Source: CAD feature listing. Evaluate the final solid. Frame: model axes, mm. Give positions to 0.01 mm unless a question says otherwise; leave off trailing zeros. Write item = value, one per line.
from build123d import *

# Parameters (mm, degrees)
ESQUISSE1_R                               = 156.21
ESQUISSE1_R_2                             = 142.07
BOSS_EXTRU_1_DEPTH                        = 2
ESQUISSE2_R                               = 5.85
ENL_V_MAT_EXTRU_1_DEPTH                   = 2
CHANFREIN1_SIZE                           = 0.5
R_P_TITION_CIRCULAIRE1_COUNT              = 70
CHANFREIN1_OF_R_P_TITION_CIRCULAIRE1_SIZE = 0.5
INTERSECT4_OUTLINE_R                      = 5.85
INTERSECT4_DEPTH                          = 2


# Read off the part's stored shape, not the designer's step: Intersect4
with BuildPart() as part:
    # Esquisse1 → Boss.-Extru.1 (new body)
    with BuildSketch(Plane(origin=(0, 0, 0), x_dir=(1, 0, 0), z_dir=(0, 1, 0))):
        with Locations(Location((0, 0, 0), (0, 0, 270))):
            Circle(ESQUISSE1_R)
        with Locations(Location((0, 0, 0), (0, 0, 270))):
            Circle(ESQUISSE1_R_2, mode=Mode.SUBTRACT)
    extrude(amount=BOSS_EXTRU_1_DEPTH)

    # Esquisse2 → Enlèv. mat.-Extru.1 (cut)
    with BuildSketch(Plane.XZ):
        with Locations(Location((-138.182447366, 56.110162301, 0), (0, 0, 270))):
            Circle(ESQUISSE2_R)
    enl_v_mat_extru_1 = extrude(amount=-ENL_V_MAT_EXTRU_1_DEPTH, mode=Mode.SUBTRACT)

    # Chanfrein1
    chanfrein1_edges = [part.edges().sort_by_distance(p)[0] for p in [
        (-138.182447366, 0, 61.960162301),
    ]]
    chamfer(chanfrein1_edges, length=CHANFREIN1_SIZE)

    # Répétition circulaire1: Enlèv. mat.-Extru.1 ×70 about axis
    r_p_tition_circulaire1_axis = Axis((0, 0, 0), (0, 1, 0))
    for i in range(1, R_P_TITION_CIRCULAIRE1_COUNT):
        add(enl_v_mat_extru_1.rotate(r_p_tition_circulaire1_axis, i * 360 / R_P_TITION_CIRCULAIRE1_COUNT), mode=Mode.SUBTRACT)

    # Chanfrein1 of Répétition circulaire1
    chanfrein1_of_r_p_tition_circulaire1_edges = [part.edges().sort_by_distance(p)[0] for p in [
        (-132.07209933, 0, 74.097307988),
        (-124.898384407, 0, 85.63786572),
        (-116.719061132, 0, 96.488917711),
        (-107.599984606, 0, 106.563097671),
        (-97.614576272, 0, 115.779294227),
        (-86.843232766, 0, 124.063303983),
        (-75.372678613, 0, 131.348428963),
        (-63.295267971, 0, 137.576013625),
        (-50.708241047, 0, 142.695917119),
        (-37.712941183, 0, 146.666916991),
        (-24.413998891, 0, 149.457041087),
        (-10.918489435, 0, 151.043824968),
        (2.664929277, 0, 151.414492782),
        (16.226891547, 0, 150.56606013),
        (29.658204426, 0, 148.505358094),
        (42.850726883, 0, 145.248978234),
        (55.698240482, 0, 140.823139006),
        (68.097304599, 0, 135.263474666),
        (79.94808926, 0, 128.614748362),
        (91.155178915, 0, 120.930491727),
        (101.628340667, 0, 112.27257388),
        (111.283250778, 0, 102.710703283),
        (120.042173586, 0, 92.321866495),
        (127.834587396, 0, 81.189708324),
        (134.597752274, 0, 69.403858359),
        (140.277215193, 0, 57.059209336),
        (144.827248457, 0, 44.255153109),
        (148.211217874, 0, 31.094780412),
        (150.40187771, 0, 17.684050826),
        (151.381590063, 0, 4.13093966),
        (151.142466863, 0, -9.455431402),
        (149.68643339, 0, -22.965672891),
        (147.02521277, 0, -36.291008285),
        (143.180231586, 0, -49.324149819),
        (138.182447366, 0, -61.960162301),
        (132.07209933, 0, -74.097307988),
        (124.898384407, 0, -85.63786572),
        (116.719061132, 0, -96.488917711),
        (107.599984606, 0, -106.563097671),
        (97.614576272, 0, -115.779294227),
        (86.843232766, 0, -124.063303983),
        (75.372678613, 0, -131.348428963),
        (63.295267971, 0, -137.576013625),
        (50.708241047, 0, -142.695917119),
        (37.712941183, 0, -146.666916991),
        (24.413998891, 0, -149.457041087),
        (10.918489435, 0, -151.043824968),
        (-2.664929277, 0, -151.414492782),
        (-16.226891547, 0, -150.56606013),
        (-29.658204426, 0, -148.505358094),
        (-42.850726883, 0, -145.248978234),
        (-55.698240482, 0, -140.823139006),
        (-68.097304599, 0, -135.263474666),
        (-79.94808926, 0, -128.614748362),
        (-91.155178915, 0, -120.930491727),
        (-101.628340667, 0, -112.27257388),
        (-111.283250778, 0, -102.710703283),
        (-120.042173586, 0, -92.321866495),
        (-127.834587396, 0, -81.189708324),
        (-134.597752274, 0, -69.403858359),
        (-140.277215193, 0, -57.059209336),
        (-144.827248457, 0, -44.255153109),
        (-148.211217874, 0, -31.094780412),
        (-150.40187771, 0, -17.684050826),
        (-151.381590063, 0, -4.13093966),
        (-151.142466863, 0, 9.455431402),
        (-149.68643339, 0, 22.965672891),
        (-147.02521277, 0, 36.291008285),
        (-143.180231586, 0, 49.324149819),
    ]]
    chamfer(chanfrein1_of_r_p_tition_circulaire1_edges, length=CHANFREIN1_OF_R_P_TITION_CIRCULAIRE1_SIZE)

    # Intersect4 outline → Intersect4 (cut)
    with BuildSketch(Plane(origin=(0, 0, 0), x_dir=(1, 0, 0), z_dir=(0, 1, 0))):
        with BuildLine():
            Line((0, 156.21), (0, 154.29748035))
            ThreePointArc((0, 154.29748035), (8.564308192, 149.115296347), (0, 143.933112344))
            Line((0, 143.933112344), (0, 142.07))
            ThreePointArc((0, 142.07), (100.458660403, -100.458660403), (-142.07, 0))
            Line((-142.07, 0), (-144.79805755, 0))
            ThreePointArc((-144.79805755, 0), (-149.086924142, -9.828457409), (-153.375790734, 0))
            Line((-153.375790734, 0), (-156.21, 0))
            ThreePointArc((-156.21, 0), (110.457150289, -110.457150289), (0, 156.21))
        make_face()
        with Locations((-89.843693539, -119.04137854)):
            Circle(INTERSECT4_OUTLINE_R, mode=Mode.SUBTRACT)
        with Locations((-78.811222339, -126.615679546)):
            Circle(INTERSECT4_OUTLINE_R, mode=Mode.SUBTRACT)
        with Locations((-118.275376678, -90.849734976)):
            Circle(INTERSECT4_OUTLINE_R, mode=Mode.SUBTRACT)
        with Locations((-125.942942241, -79.881877626)):
            Circle(INTERSECT4_OUTLINE_R, mode=Mode.SUBTRACT)
        with Locations((-100.152796146, -110.50862635)):
            Circle(INTERSECT4_OUTLINE_R, mode=Mode.SUBTRACT)
        with Locations((-109.655527327, -101.086123678)):
            Circle(INTERSECT4_OUTLINE_R, mode=Mode.SUBTRACT)
        with Locations((-54.936591001, -138.653200622)):
            Circle(INTERSECT4_OUTLINE_R, mode=Mode.SUBTRACT)
        with Locations((-42.286655355, -143.019501651)):
            Circle(INTERSECT4_OUTLINE_R, mode=Mode.SUBTRACT)
        with Locations((-67.144209517, -133.170545549)):
            Circle(INTERSECT4_OUTLINE_R, mode=Mode.SUBTRACT)
        with Locations((-29.296252425, -146.234293746)):
            Circle(INTERSECT4_OUTLINE_R, mode=Mode.SUBTRACT)
        with Locations((-16.069973297, -148.271693292)):
            Circle(INTERSECT4_OUTLINE_R, mode=Mode.SUBTRACT)
        with Locations((-2.714308192, -149.115296347)):
            Circle(INTERSECT4_OUTLINE_R, mode=Mode.SUBTRACT)
        with Locations((-132.596489287, -68.270858368)):
            Circle(INTERSECT4_OUTLINE_R, mode=Mode.SUBTRACT)
        with Locations((-138.182447366, -56.110162301)):
            Circle(INTERSECT4_OUTLINE_R, mode=Mode.SUBTRACT)
        with Locations((-142.655841629, -43.497700199)):
            Circle(INTERSECT4_OUTLINE_R, mode=Mode.SUBTRACT)
        with Locations((-145.980654936, -30.535020192)):
            Circle(INTERSECT4_OUTLINE_R, mode=Mode.SUBTRACT)
        with Locations((-148.130117844, -17.326490156)):
            Circle(INTERSECT4_OUTLINE_R, mode=Mode.SUBTRACT)
        with Locations((10.663210926, -148.758310713)):
            Circle(INTERSECT4_OUTLINE_R, mode=Mode.SUBTRACT)
        with Locations((23.95487614, -147.20361063)):
            Circle(INTERSECT4_OUTLINE_R, mode=Mode.SUBTRACT)
        with Locations((37.053670776, -144.463713629)):
            Circle(INTERSECT4_OUTLINE_R, mode=Mode.SUBTRACT)
        with Locations((49.854131043, -140.560679749)):
            Circle(INTERSECT4_OUTLINE_R, mode=Mode.SUBTRACT)
        with Locations((62.25319516, -135.525933924)):
            Circle(INTERSECT4_OUTLINE_R, mode=Mode.SUBTRACT)
        with Locations((74.151033153, -129.400012967)):
            Circle(INTERSECT4_OUTLINE_R, mode=Mode.SUBTRACT)
        with Locations((85.451850628, -122.232239191)):
            Circle(INTERSECT4_OUTLINE_R, mode=Mode.SUBTRACT)
        with Locations((96.064660047, -114.080323297)):
            Circle(INTERSECT4_OUTLINE_R, mode=Mode.SUBTRACT)
        with Locations((105.904013308, -105.009899718)):
            Circle(INTERSECT4_OUTLINE_R, mode=Mode.SUBTRACT)
        with Locations((114.890689725, -95.093998171)):
            Circle(INTERSECT4_OUTLINE_R, mode=Mode.SUBTRACT)
        with Locations((122.952333862, -84.412455665)):
            Circle(INTERSECT4_OUTLINE_R, mode=Mode.SUBTRACT)
        with Locations((130.024038102, -73.0512737)):
            Circle(INTERSECT4_OUTLINE_R, mode=Mode.SUBTRACT)
        with Locations((136.04886524, -61.101925832)):
            Circle(INTERSECT4_OUTLINE_R, mode=Mode.SUBTRACT)
        with Locations((140.97830691, -48.660621186)):
            Circle(INTERSECT4_OUTLINE_R, mode=Mode.SUBTRACT)
        with Locations((144.772674148, -35.827529829)):
            Circle(INTERSECT4_OUTLINE_R, mode=Mode.SUBTRACT)
        with Locations((147.401416938, -22.705976268)):
            Circle(INTERSECT4_OUTLINE_R, mode=Mode.SUBTRACT)
        with Locations((148.843370189, -9.401607537)):
            Circle(INTERSECT4_OUTLINE_R, mode=Mode.SUBTRACT)
        with Locations((149.086924142, 3.978457409)):
            Circle(INTERSECT4_OUTLINE_R, mode=Mode.SUBTRACT)
        with Locations((148.130117844, 17.326490156)):
            Circle(INTERSECT4_OUTLINE_R, mode=Mode.SUBTRACT)
        with Locations((145.980654936, 30.535020192)):
            Circle(INTERSECT4_OUTLINE_R, mode=Mode.SUBTRACT)
        with Locations((142.655841629, 43.497700199)):
            Circle(INTERSECT4_OUTLINE_R, mode=Mode.SUBTRACT)
        with Locations((138.182447366, 56.110162301)):
            Circle(INTERSECT4_OUTLINE_R, mode=Mode.SUBTRACT)
        with Locations((132.596489287, 68.270858368)):
            Circle(INTERSECT4_OUTLINE_R, mode=Mode.SUBTRACT)
        with Locations((16.069973297, 148.271693292)):
            Circle(INTERSECT4_OUTLINE_R, mode=Mode.SUBTRACT)
        with Locations((29.296252425, 146.234293746)):
            Circle(INTERSECT4_OUTLINE_R, mode=Mode.SUBTRACT)
        with Locations((67.144209517, 133.170545549)):
            Circle(INTERSECT4_OUTLINE_R, mode=Mode.SUBTRACT)
        with Locations((42.286655355, 143.019501651)):
            Circle(INTERSECT4_OUTLINE_R, mode=Mode.SUBTRACT)
        with Locations((54.936591001, 138.653200622)):
            Circle(INTERSECT4_OUTLINE_R, mode=Mode.SUBTRACT)
        with Locations((109.655527327, 101.086123678)):
            Circle(INTERSECT4_OUTLINE_R, mode=Mode.SUBTRACT)
        with Locations((100.152796146, 110.50862635)):
            Circle(INTERSECT4_OUTLINE_R, mode=Mode.SUBTRACT)
        with Locations((125.942942241, 79.881877626)):
            Circle(INTERSECT4_OUTLINE_R, mode=Mode.SUBTRACT)
        with Locations((118.275376678, 90.849734976)):
            Circle(INTERSECT4_OUTLINE_R, mode=Mode.SUBTRACT)
        with Locations((78.811222339, 126.615679546)):
            Circle(INTERSECT4_OUTLINE_R, mode=Mode.SUBTRACT)
        with Locations((89.843693539, 119.04137854)):
            Circle(INTERSECT4_OUTLINE_R, mode=Mode.SUBTRACT)
    extrude(amount=INTERSECT4_DEPTH, mode=Mode.SUBTRACT)


solid = part.part
1) Material intervals for L1, parallel to X at y = 1.6, z = -97; L2, parallel to X at y = 0.6, z = -114; L3, parallel to X at y = 0.6, z = -130.5, sorted ascending.
Computed:
L1 = -122.44 to -120.42, -109.36 to -103.8
L2 = -106.8 to -101.91, -90.22 to -84.78
L3 = -85.86 to -79.9, -68.41 to -65.25, -59.26 to -56.16
2) Draft query along X for faces 1 (the flat face through (-95, 0, -107)), 2 (the cylindrical face through (-109.2, 1, -111.7)), 3 (the cylindrical face through (-67.051, 1.24, -138.874)). Return one class per face: pulls with the +X half, pulls with the -X half, needs draft (parallel to the pull), parting line crosses it, or undercut.
Computed:
face_1 = needs draft
face_2 = pulls with the -X half
face_3 = undercut
3) Cut plane A-A (y = 1.4). State how many separate pieces and enclosed holes the cut face has, then the cut area to 3 significant figures.
Computed:
separate_pieces = 1
enclosed_holes = 17
area = 1,450 mm²
4) Contact query for flat-ended pins moving along their axis: pin 1 (1 mm diameter, centred on y = 1.5, z = -24, fed in from -X); pin 2 (7 mm diameter, centred on x = -49.85, z = -140.56, fed in from +Y). Output: stop coordinate, or through.
Computed:
pin_1 = -154.43
pin_2 = through
